Read the model definition and answer for the solid it produces. Units are mm, in the model's axes. A direction names the side the tool comes from. Coordinates: 2 decimals unless noted, no trailing zeros. Write each loop counter-clockwise with the first axis right and the second up, starting at its lowest first coordinate (ties: lowest second). Pieces come first, ordered by that corner, then holes.
from build123d import *

# Parameters (mm, degrees)
CROQUIS1_W              = 44
CROQUIS1_H              = 5
SALIENTE_EXTRUIR1_DEPTH = 10
CROQUIS2_R              = 2
SALIENTE_EXTRUIR2_DEPTH = 5


with BuildPart() as part:
    # Croquis1 → Saliente-Extruir1 (new body)
    with BuildSketch(Plane.XY):
        Rectangle(CROQUIS1_W, CROQUIS1_H)
    extrude(amount=SALIENTE_EXTRUIR1_DEPTH)

    # Croquis2 → Saliente-Extruir2 (add)
    with BuildSketch(Plane.XY.offset(10)):
        with Locations(Location((-20, 0, 0), (0, 0, 180))):
            Circle(CROQUIS2_R)
        with Locations((20, 0)):
            Circle(CROQUIS2_R)
    extrude(amount=SALIENTE_EXTRUIR2_DEPTH)


solid = part.part
Item 1: The part is cut by section C-C (x = 20). Give the vertices of the cut face in (y, z).
Item 2: The part is cut by section B-B (y = -1.2). Give the vertices of the cut face in (x, z), and give its area (3 significant figures).
Item 3: Given pin 1 (3 mm diameter, centred on y = -1.5, z = 11.5, fed in from -X), flat-ended and moving along its own axis, determine where the tip first touches the part or whether it passes through.
Item 4: The part is cut by section D-D (y = 0.5). Give the vertices of the cut face in (x, z).
Item 5: For faces 1 (the flat face through (0, -2.5, 5)), 2 (the cylindrical face through (-18.4, 1.2, 12.5)), determine the directions among +Z, -Z, +X, -X, +Y, -Y from which every point of the face is accessible in a straight line to the end or side of a thin tool.
Item 6: The part is cut by section A-A (z = 13.75). Give the vertices of the cut face in (x, y).
Item 7: Find the intervals of material crossed by probe 1 along Z at (x, y) = (4, 1.7); probe 2 along X at (y, z) = (-1.25, 12); probe 3 along X at (y, z) = (0.4, 13), in increasing order.
Answer:
1. outline: (-2.5, 0) - (2.5, 0) - (2.5, 10) - (2, 10) - (2, 15) - (-2, 15) - (-2, 10) - (-2.5, 10) - close
2. outline: (-22, 0) - (22, 0) - (22, 10) - (21.6, 10) - (21.6, 15) - (18.4, 15) - (18.4, 10) - (-18.4, 10) - (-18.4, 15) - (-21.6, 15) - (-21.6, 10) - (-22, 10) - close
2. area: 472 mm2
3. pin 1: stops at x = -22
4. outline: (-22, 0) - (22, 0) - (22, 10) - (21.94, 10) - (21.94, 15) - (18.06, 15) - (18.06, 10) - (-18.06, 10) - (-18.06, 15) - (-21.94, 15) - (-21.94, 10) - (-22, 10) - close
5. face 1: +Z, -Z, +X, -X, -Y
5. face 2: +Z
6. outline: circle Ø4 at (-20, 0); circle Ø4 at (20, 0)
7. probe 1: z = 0 to 10
7. probe 2: x = -21.56 to -18.44, 18.44 to 21.56
7. probe 3: x = -21.96 to -18.04, 18.04 to 21.96
